Could you check a few things on this model? Use its own coordinates, in mm. A direction names the side the tool comes from. Give positions to 0.01 mm unless a question says otherwise; leave off trailing zeros. Loops run counter-clockwise (first coordinate to the right, second up) from the corner with the lowest first, then second, coordinate; pieces in that order, holes last. Notation, with made-up numbers: (51.25, 88.25) -> (108.25, 88.25) arc R18 ccw to (108.25, 110.25) -> close; hole circle Ø5 at (10.25, 11.25). An arc over 180 degrees is marked (long way). Write item = value, one per line. Start each with the question number.
1) I want a section at A-A (z = 1.5). List the corners of the cut face in (x, y) for me (1 decimal), and give its area (3 significant figures).
2) I'm going to push flat-ended pins straight in: pin 1 Ø6 at (x, z) = (3, 3.5) entering from -Y; pin 2 Ø0.9 at (y, z) = (2.5, 15) entering from -X; pin 3 Ø0.7 at (x, z) = (-5, 11) entering from -Y. Where does each tip first touch, or does it pass through?
3) I want a section at B-B (y = 0). List the corners of the cut face in (x, z) for me, and give its area (3 significant figures).
4) I want a section at C-C (y = 8.5). List the corners of the cut face in (x, z) for me, and give its area (3 significant figures).
5) If we mould it in two halves opening along X, with no side actions, what happens to faces 1 (the face through (-18.83, 6.09, 12.32)), 2 (the face through (-6, 6, 12)), 3 (the face through (18.452, 6.167, 12.325))? For each: +X half, -X half, draft (parallel to the pull), parting line (faces both ways), or undercut.
6) I want a section at D-D (x = -23). List the corners of the cut face in (y, z) for me.
7) I need wall thicknesses on probe 1 along X at (y, z) = (10, 1.5); probe 2 along X at (y, z) = (8, 6); probe 3 along Y at (x, z) = (-3, 18.5). Which ranges of each line are inside material? Lowest first, please. Write a range as from..to.
8) On a 3-axis mill with a long thin cutter (end or side, diameter ignored), from which of +Z, -Z, +X, -X, +Y, -Y can I reach the whole of each face in a straight line? I mean faces 4 (the face through (-5, 9, 12)), 5 (the face through (5, 2, 12)), 6 (the face through (-0.07, 9.533, 12.325)). Say none if no direction works.
Autodesk Inventor part; units mm, degrees
ref_plane "YZ Plane" through (0, 0, 0) normal (1, 0, 0) x (0, 1, 0)
ref_plane "XZ Plane" through (0, 0, 0) normal (0, 1, 0) x (-1, 0, 0)
ref_plane "XY Plane" through (0, 0, 0) normal (0, 0, 1) x (1, 0, 0)
sketch "Sketch1" plane through (0, 0, 0) normal (0, 0, 1) x (1, 0, 0)
  arc A0 (31, 0) -> (-31, 0) centre (0, -84.0628) ccw construction
  arc A1 (31.865, 2.3456) -> (-31.865, 2.3456) centre (0, -84.0628) ccw
  arc A2 (30.135, -2.3456) -> (-30.135, -2.3456) centre (0, -84.0628) ccw
  arc A3 (30.135, -2.3456) -> (31.865, 2.3456) centre (31, 0) ccw
  arc A4 (-31.865, 2.3456) -> (-30.135, -2.3456) centre (-31, 0) ccw
  line L0 (5, 0.5338) -> (5, 10.5338)
  line L1 (5, 10.5338) -> (-5, 10.5338)
  line L2 (-5, 10.5338) -> (-5, 0.5338)
  line L3 (-5, 0.5338) -> (5, 10.5338) construction
  line L4 (5, 0.5338) -> (-5, 10.5338) construction
  circle A5 centre (0, 5.5338) radius 4
  line L5 (-6, 4.2838) -> (6, 4.2838)
  line L6 (6, 4.2838) -> (6, 6.7838)
  line L7 (6, 6.7838) -> (-6, 6.7838)
  line L8 (-6, 6.7838) -> (-6, 4.2838)
  arc A6 (5, 0.5338) -> (-5, 0.5338) centre (0, -20.4862) ccw
  point P0 (0, 0)
  point P1 (3.7997, 4.2838)
  point P2 (-3.7997, 4.2838)
  point P3 (-3.7997, 6.7838)
  point P4 (3.7997, 6.7838)
  point P5 (5, 2.8902)
  point P6 (5, 7.898)
  point P7 (-5, 7.898)
  point P8 (-5, 2.8902)
  point P9 (3.0781, 2.9794)
  point P10 (-3.0781, 2.9794)
  dimension "d0" = 62
  dimension "d1" = 5
  dimension "d2" = 87.0966
  dimension "d3" = 10
  dimension "d4" = 10
  dimension "d5" = 8
  dimension "d6" = 12
  dimension "d7" = 2.5
  dimension "d8" = 1.25
extrude "Extrusion1" add sketch "Sketch1" along normal blind 25 contours A3 A2 L0 L5 L6 L7 A1 | L0 L7 A5 A1 | A1 A5 L2 L1 L0 | L0 A6 L2 A2 A5 | A2 A5 L5 L0 | A5 L7 L2 A1 | L2 L7 L8 L5 A2 A4 A1 | A2 L2 L5 A5
fillet "Fillet2" radius 1 1 edges at (5, 0.5338, 12.5)
fillet "Fillet3" radius 1 1 edges at (-5, 0.5338, 12.5)
properties part number "sorter_3DPrint"
Answer list:
q1.outline = (-31.9, 2.3) arc R2.5 ccw to (-30.1, -2.3) arc R87.1 cw to (-5, 2.9) -> (-5, 1.8) arc R1 ccw to (-3.8, 0.8) arc R21.6 cw to (3.8, 0.8) arc R1 ccw to (5, 1.8) -> (5, 2.9) arc R87.1 cw to (30.1, -2.3) arc R2.5 ccw to (31.9, 2.3) arc R92.1 ccw to (5, 7.9) -> (5, 10.5) -> (-5, 10.5) -> (-5, 7.9) arc R92.1 ccw to start; hole (-6, 4.3) -> (-3.8, 4.3) arc R4 ccw to (3.8, 4.3) -> (6, 4.3) -> (6, 6.8) -> (3.8, 6.8) arc R4 ccw to (-3.8, 6.8) -> (-6, 6.8) -> close
q1.area = 321 mm^2
q2.pin_1 = 0.76
q2.pin_2 = -32.43
q2.pin_3 = 1
q3.outline = (-33.5, 0) -> (-22.79, 0) -> (-22.79, 25) -> (-33.5, 25) -> close; (22.79, 0) -> (33.5, 0) -> (33.5, 25) -> (22.79, 25) -> close
q3.area = 536 mm^2
q4.outline = (-5, 0) -> (-2.68, 0) -> (-2.68, 25) -> (-5, 25) -> close; (2.68, 0) -> (5, 0) -> (5, 25) -> (2.68, 25) -> close
q4.area = 116 mm^2
q5.face_1 = -X half
q5.face_2 = undercut
q5.face_3 = +X half
q6.outline = (-0.06, 0) -> (5.12, 0) -> (5.12, 25) -> (-0.06, 25) -> close
q7.probe_1 = -5..5
q7.probe_2 = -5..-3.15, 3.15..5
q7.probe_3 = 0.91..2.89, 8.18..10.53
q8.face_4 = +Z, -Z, -X, +Y
q8.face_5 = +Z, -Z, -Y
q8.face_6 = +Z, -Z
